Here's the drawing with two shaded views (mm, measured from the low corner). I have some questions. Round coordinates to 2 decimals unless told otherwise and drop trailing zeros. Write each loop counter-clockwise with the first axis right and the second up, starting at its lowest first coordinate (ties: lowest second). Pieces come first, ordered by that corner, then holes. Notation, with made-up numbers: M -2.5,51.5 L 48.5,51.5 A14 ccw 48.5,72.5 Z; hole C -32.75,58 d6. An arc over 180 degrees is marked long. Write item = value, one per line. Start each with the question number.
(1) I want a section at D-D (y = 1.3). Give the number of separate pieces and of enclosed holes in the cut face, and give its area (3 significant figures).
(2) Will these pins go through, and if not, where does the flat tip stop? pin 1 Ø4.5 at (x, z) = (5, 40) entering from -Y; pin 2 Ø3 at (x, z) = (5, 5) entering from +Y.
(3) I want a section at A-A (z = 5). List the corners of the cut face in (x, y) for me.
(4) I want a section at C-C (x = 30). List the corners of the cut face in (y, z) for me, and give its area (4 significant figures).
(5) I need wall thicknesses on line 1 along Z through (x, y) = (21.25, 1.9); line 2 along Z through (x, y) = (55, 1.4); line 3 along X through (y, z) = (1.7, 39). Which ranges of each line are inside material? Lowest first, please.
(6) I want a section at B-B (x = 5). List the corners of the cut face in (y, z) for me.
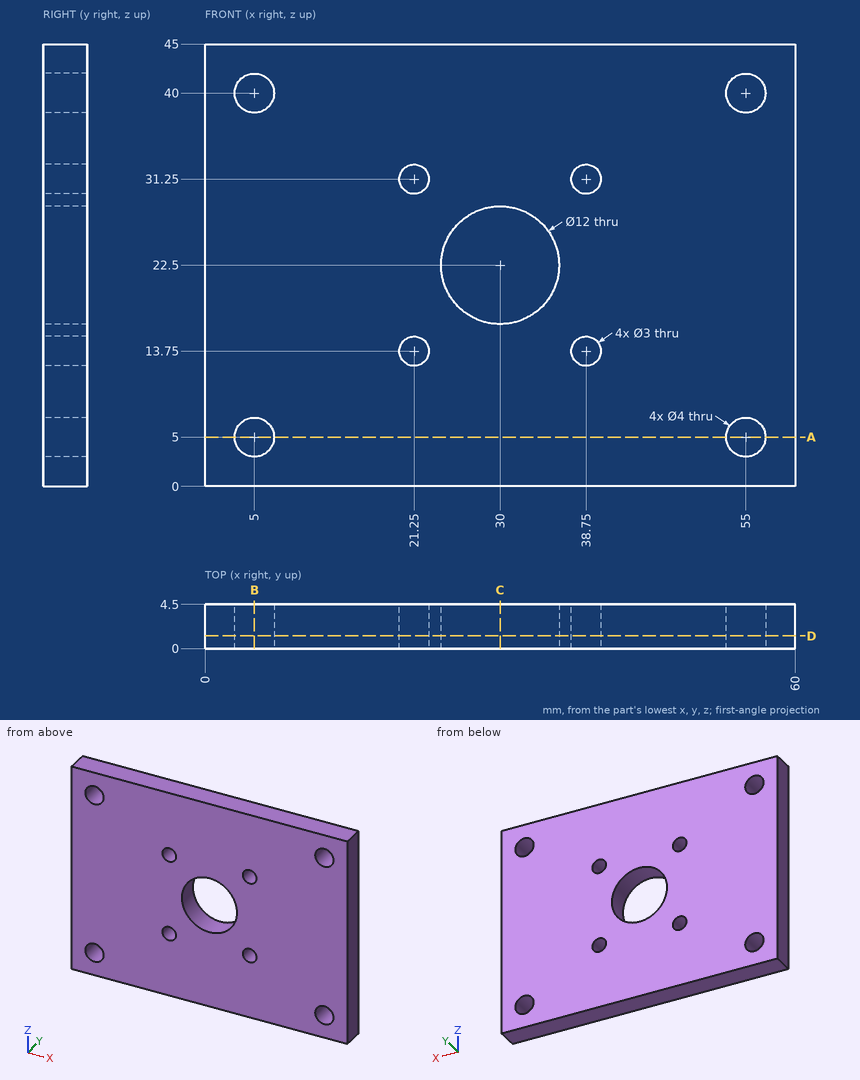
Returned:
q1.separate_pieces = 1
q1.enclosed_holes = 9
q1.area = 2,510 mm²
q2.pin_1 = 0
q2.pin_2 = through
q3.outline = M 0,0 L 3,0 L 3,4.5 L 0,4.5 Z; M 7,0 L 53,0 L 53,4.5 L 7,4.5 Z; M 57,0 L 60,0 L 60,4.5 L 57,4.5 Z
q4.outline = M 0,0 L 4.5,0 L 4.5,16.5 L 0,16.5 Z; M 0,28.5 L 4.5,28.5 L 4.5,45 L 0,45 Z
q4.area = 148.5 mm²
q5.line_1 = 0 to 12.25, 15.25 to 29.75, 32.75 to 45
q5.line_2 = 0 to 3, 7 to 38, 42 to 45
q5.line_3 = 0 to 3.27, 6.73 to 53.27, 56.73 to 60
q6.outline = M 0,0 L 4.5,0 L 4.5,3 L 0,3 Z; M 0,7 L 4.5,7 L 4.5,38 L 0,38 Z; M 0,42 L 4.5,42 L 4.5,45 L 0,45 Z
